Autodesk Fusion 360 part; units mm, degrees
sketch "Sketch1" plane through (0, 0, 0) normal (0, 0, 1) x (1, 0, 0)
  line L0 (0, 0) -> (322, 0)
  line L1 (322, 0) -> (322, 322)
  line L2 (322, 322) -> (0, 322)
  line L3 (0, 322) -> (0, 0)
  dimension "d1" = 322
  dimension "d2" = 322
extrude "Extrude1" add sketch "Sketch1" against normal blind 11
sketch "Sketch2" plane through (0, 0, -11) normal (0, 0, -1) x (1, 0, 0)
  line L0 (0, 0) -> (0, -322)
  line L1 (0, -322) -> (322, -322)
  line L2 (322, -322) -> (322, 0)
  line L3 (322, 0) -> (0, 0)
  line L4 (41, -41) -> (279.137, -41)
  line L5 (279.137, -41) -> (279.137, -280.7037)
  line L6 (279.137, -280.7037) -> (41, -280.7037)
  line L7 (41, -280.7037) -> (41, -41)
  dimension "d7" = 41
  dimension "d8" = 41
extrude "Extrude2" add sketch "Sketch2" along normal blind 30 contours L4 L5 L6 L7
For this review, take the finished solid that the model builds, in its own axes (mm). A direction names the side the tool comes from. Round coordinates to 2 decimals unless told otherwise and drop trailing zeros. Write each loop counter-clockwise with the first axis right and the second up, starting at its lowest first coordinate (ties: lowest second). Pieces come first, ordered by that corner, then holes. Notation, with made-up numbers: M 37,65.25 L 48,65.25 A31 cw 48,100.25 Z; hole C 74.25,67.25 d10. An arc over 180 degrees is marked long. Write item = value, one per line. Start each with the question number.
(1) For faces 1 (the face through (162, 280.704, -26)), 2 (the face through (279.137, 159, -26)), 3 (the face through (158, 41, -26)), list the 3-axis set-ups (+Z, -Z, +X, -X, +Y, -Y) from which the entire face can be reached by the end or side of a thin tool; tool diameter is ignored.
(2) Clearance check with flat-ended pins moving along their axes: pin 1 Ø9 at (y, z) = (181.5, -23) entering from -X; pin 2 Ø15 at (x, z) = (187, -28) entering from -Y; pin 3 Ø9 at (y, z) = (121, -21.5) entering from +X. State where each tip first meets the part, or that it passes through.
(3) We need section C-C (z = -30.5). Give the boundary of the cut face in (x, y), then the cut area to 3 significant figures.
(4) We need section B-B (x = 247.5). Give the boundary of the cut face in (y, z).
(5) We need section A-A (y = 85.5). Give the boundary of the cut face in (x, z).
(6) We need section D-D (x = 286). Give the boundary of the cut face in (y, z), then the cut area to 3 significant figures.
(7) For line 1 along X through (y, z) = (231, -24); line 2 along Y through (x, z) = (240.5, -19); line 3 along Z through (x, y) = (62, 21), list the stretches that pass through material, from the lowest coordinate up.
Results found:
q1.face_1 = -Z, +X, -X, +Y
q1.face_2 = -Z, +X, +Y, -Y
q1.face_3 = -Z, +X, -X, -Y
q2.pin_1 = 41
q2.pin_2 = 41
q2.pin_3 = 279.14
q3.outline = M 41,41 L 279.14,41 L 279.14,280.7 L 41,280.7 Z
q3.area = 57,100 mm²
q4.outline = M 0,-11 L 41,-11 L 41,-41 L 280.7,-41 L 280.7,-11 L 322,-11 L 322,0 L 0,0 Z
q5.outline = M 0,-11 L 41,-11 L 41,-41 L 279.14,-41 L 279.14,-11 L 322,-11 L 322,0 L 0,0 Z
q6.outline = M 0,-11 L 322,-11 L 322,0 L 0,0 Z
q6.area = 3,540 mm²
q7.line_1 = 41 to 279.14
q7.line_2 = 41 to 280.7
q7.line_3 = -11 to 0
